For this review, take the finished solid that the model builds, in its own axes (mm). A direction names the side the tool comes from. Coordinates: 2 decimals unless noted, no trailing zeros. Write each loop counter-clockwise with the first axis right and the second up, starting at its lowest first coordinate (ties: lowest second). Pieces come first, ordered by that corner, then holes.
1) Insertion check: P1, Ø6, axis at x = 13.5, y = 476, coming from the -Z side; P2, Ø4, axis at x = 1.5, y = 165.5, coming from the -Z side; P3, Ø3.5, axis at y = 117.48, z = -28.98, coming from the -X side; P4, Ø5.5, axis at x = 91, z = -25, coming from the -Y side. Each pin has a flat end and moves straight along its axis. Give the tip position at first contact, or say it passes through.
2) We need section A-A on y = 508. Write out the cut boundary in (x, z), then the cut area to 3 significant figures.
3) We need section C-C on x = 23. Write out the cut boundary in (y, z).
4) To check wall thickness, follow line 1 along Y through (x, z) = (64, -3); line 2 along Z through (x, y) = (53, 351); line 3 along X through (y, z) = (61.5, -31). State the ranges of each line that lie inside material, in increasing order.
5) For faces 4 (the face through (95, 603.25, -16)), 5 (the face through (94.4, 358.6, -24.9)), 6 (the face through (51, 609.6, -2)), 7 (the face through (97.028, 59, -20)), list the 3-axis set-ups (+Z, -Z, +X, -X, +Y, -Y) from which the entire face can be reached by the end or side of a thin tool; tool diameter is ignored.
6) Mouldability with a two-part tool opening along X and no side actions: class faces 1 (the face through (52, 368, 0)), 2 (the face through (7.13, 358.57, -25.31)), 3 (the face through (0, 301, -20)) as pulls with the +X half, pulls with the -X half, needs draft (parallel to the pull), parting line crosses it, or undercut.
7) We need section B-B on y = 223.5. Write out the cut boundary in (x, z), then the cut area to 3 significant figures.
from build123d import *

# Parameters (mm, degrees)
BOSS_EXTRUDE1_DEPTH = 609.6
SKETCH5_W           = 92.456
SKETCH5_H           = 40.132
CUT_EXTRUDE4_DEPTH  = 94.488
SKETCH6_R           = 3.0734
SKETCH6_W           = 45.116342256
SKETCH6_H           = 16.485642943
SKETCH6_W_2         = 12.7
SKETCH6_H_2         = 20.2565
CUT_EXTRUDE5_DEPTH  = 620.310340156
SKETCH4_R           = 4.064
SKETCH4_W           = 3.175
SKETCH4_H           = 82.55
SKETCH4_R_2         = 1.524
CUT_EXTRUDE3_DEPTH  = 620.310340156
SKETCH7_W           = 92.456
SKETCH7_H           = 35.3314
CUT_EXTRUDE6_DEPTH  = 6.35
SKETCH8_W           = 92.456
SKETCH8_H           = 35.3314
CUT_EXTRUDE7_DEPTH  = 26.162
SKETCH10_R          = 1.1303
CUT_EXTRUDE8_DEPTH  = 12.7
CHAMFER1_SIZE       = 1.905
FILLET1_R           = 3.175


with BuildPart() as part:
    # Sketch1 → Boss-Extrude1 (new body)
    with BuildSketch(Plane(origin=(0, 0, 0), x_dir=(1, 0, 0), z_dir=(0, 1, 0))):
        with BuildLine():
            Line((0, 0), (0, 40.132))
            Line((0, 40.132), (2.032, 40.132))
            Line((2.032, 40.132), (4.572, 40.132))
            Line((4.572, 40.132), (9.758667803, 10.070937859))
            ThreePointArc((9.758667803, 10.070937859), (11.925571203, 6.293730916), (16.016209625, 4.8006))
            Line((16.016209625, 4.8006), (85.583790375, 4.8006))
            ThreePointArc((85.583790375, 4.8006), (89.674428797, 6.293730916), (91.841332197, 10.070937859))
            Line((91.841332197, 10.070937859), (97.028, 40.132))
            Line((97.028, 40.132), (99.568, 40.132))
            Line((99.568, 40.132), (101.6, 40.132))
            Line((101.6, 40.132), (101.6, 0))
            Line((101.6, 0), (0, 0))
        make_face()
    extrude(amount=BOSS_EXTRUDE1_DEPTH)

    # Sketch5 → Cut-Extrude4 (cut)
    with BuildSketch(Plane.XZ):
        with Locations((50.8, -20.066)):
            Rectangle(SKETCH5_W, SKETCH5_H)
    extrude(amount=-CUT_EXTRUDE4_DEPTH, mode=Mode.SUBTRACT)

    # Sketch6 → Cut-Extrude5 (cut, through all)
    with BuildSketch(Plane.XY):
        with Locations((39.7891, 596.796653012)):
            Circle(SKETCH6_R)
        with Locations((39.7891, 556.283653012)):
            Circle(SKETCH6_R)
        with Locations((61.8109, 556.283653012)):
            Circle(SKETCH6_R)
        with Locations((61.8109, 596.796653012)):
            Circle(SKETCH6_R)
        with Locations((50.8, 102.730821472)):
            Rectangle(SKETCH6_W, SKETCH6_H)
        with Locations((77.5081, 586.668403012)):
            Rectangle(SKETCH6_W_2, SKETCH6_H_2)
    extrude(amount=-CUT_EXTRUDE5_DEPTH, mode=Mode.SUBTRACT)

    # Sketch4 → Cut-Extrude3 (cut, through all)
    with BuildSketch(Plane.ZY):
        with BuildLine():
            Line((-25.208591254, 24.104081866), (-25.208591254, 29.184081866))
            ThreePointArc((-25.208591254, 29.184081866), (-29.971091254, 33.946581866), (-34.733591254, 29.184081866))
            Line((-34.733591254, 29.184081866), (-34.733591254, 24.104081866))
            ThreePointArc((-34.733591254, 24.104081866), (-29.971091254, 19.341581866), (-25.208591254, 24.104081866))
        make_face()
        with Locations((-20.066, 69.088)):
            Circle(SKETCH4_R)
        with Locations((-38.5445, 155.575)):
            Rectangle(SKETCH4_W, SKETCH4_H)
        with Locations((-38.5445, 320.675)):
            Rectangle(SKETCH4_W, SKETCH4_H)
        with Locations((-38.5445, 485.775)):
            Rectangle(SKETCH4_W, SKETCH4_H)
        with Locations(Location((-28.9814, 117.475, 0), (0, 0, 180))):
            Circle(SKETCH4_R_2)
        with Locations((-11.1506, 117.475)):
            Circle(SKETCH4_R_2)
        with Locations(Location((-11.1506, 606.425, 0), (0, 0, 315.108108431))):
            Circle(SKETCH4_R_2)
        with Locations((-28.9814, 606.425)):
            Circle(SKETCH4_R_2)
    extrude(amount=-CUT_EXTRUDE3_DEPTH, mode=Mode.SUBTRACT)

    # Sketch7 → Cut-Extrude6 (cut)
    with BuildSketch(Plane(origin=(0, 609.6, 0), x_dir=(1, 0, 0), z_dir=(0, 1, 0))):
        with Locations((50.8, 22.4663)):
            Rectangle(SKETCH7_W, SKETCH7_H)
    extrude(amount=-CUT_EXTRUDE6_DEPTH, mode=Mode.SUBTRACT)

    # Sketch8 → Cut-Extrude7 (cut)
    with BuildSketch(Plane.XZ.offset(-94.488)):
        with Locations((50.8, -22.4663)):
            Rectangle(SKETCH8_W, SKETCH8_H)
    extrude(amount=-CUT_EXTRUDE7_DEPTH, mode=Mode.SUBTRACT)

    # Sketch10 → Cut-Extrude8 (cut)
    with BuildSketch(Plane(origin=(0, 0, -36.957), x_dir=(-1, 0, 0), z_dir=(0, 0, -1))):
        with Locations((-2.286, 155.321)):
            Circle(SKETCH10_R)
        with Locations((-2.286, 320.421)):
            Circle(SKETCH10_R)
        with Locations((-2.286, 485.64141222)):
            Circle(SKETCH10_R)
        with Locations((-99.314, 155.321)):
            Circle(SKETCH10_R)
        with Locations((-99.314, 320.421)):
            Circle(SKETCH10_R)
        with Locations((-99.314, 485.64141222)):
            Circle(SKETCH10_R)
    extrude(amount=-CUT_EXTRUDE8_DEPTH, mode=Mode.SUBTRACT)

    # Chamfer1
    # the kernel refuses this chamfer: 1.905 mm, written as the material it takes off along each edge
    with BuildSketch(Plane(origin=(0, 117.475, -28.9814), x_dir=(0, 0, -1), z_dir=(0, 1, 0))) as chamfer1_piece_1:
        Polygon((1.524, -CHAMFER1_SIZE), (1.524 + CHAMFER1_SIZE, 0), (1.524, 0), align=None)
    revolve(axis=Axis((0, 117.475, -28.9814), (-1, 0, 0)), mode=Mode.SUBTRACT)
    with BuildSketch(Plane(origin=(101.6, 117.475, -28.9814), x_dir=(0, 0, -1), z_dir=(0, 1, 0))) as chamfer1_piece_2:
        Polygon((1.524, CHAMFER1_SIZE), (1.524 + CHAMFER1_SIZE, 0), (1.524, 0), align=None)
    revolve(axis=Axis((101.6, 117.475, -28.9814), (-1, 0, 0)), mode=Mode.SUBTRACT)
    with BuildSketch(Plane(origin=(101.6, 117.475, -11.1506), x_dir=(0, 0, 1), z_dir=(0, -1, 0))) as chamfer1_piece_3:
        Polygon((1.524, CHAMFER1_SIZE), (1.524 + CHAMFER1_SIZE, 0), (1.524, 0), align=None)
    revolve(axis=Axis((101.6, 117.475, -11.1506), (-1, 0, 0)), mode=Mode.SUBTRACT)
    with BuildSketch(Plane(origin=(0, 117.475, -11.1506), x_dir=(0, 0, 1), z_dir=(0, -1, 0))) as chamfer1_piece_4:
        Polygon((1.524, -CHAMFER1_SIZE), (1.524 + CHAMFER1_SIZE, 0), (1.524, 0), align=None)
    revolve(axis=Axis((0, 117.475, -11.1506), (-1, 0, 0)), mode=Mode.SUBTRACT)
    with BuildSketch(Plane(origin=(0, 606.425, -11.1506), x_dir=(0, -0.7057713201939051, 0.7084397247414577), z_dir=(0, -0.7084397247414577, -0.7057713201939051))) as chamfer1_piece_5:
        Polygon((1.524, -CHAMFER1_SIZE), (1.524 + CHAMFER1_SIZE, 0), (1.524, 0), align=None)
    revolve(axis=Axis((0, 606.425, -11.1506), (-1, 0, 0)), mode=Mode.SUBTRACT)
    with BuildSketch(Plane(origin=(101.6, 606.425, -11.1506), x_dir=(0, -0.7057713201939051, 0.7084397247414577), z_dir=(0, -0.7084397247414577, -0.7057713201939051))) as chamfer1_piece_6:
        Polygon((1.524 + CHAMFER1_SIZE, 0), (1.524, CHAMFER1_SIZE), (1.524, 0), align=None)
    revolve(axis=Axis((101.6, 606.425, -11.1506), (-1, 0, 0)), mode=Mode.SUBTRACT)
    with BuildSketch(Plane(origin=(101.6, 606.425, -28.9814), x_dir=(0, 0, 1), z_dir=(0, -1, 0))) as chamfer1_piece_7:
        Polygon((1.524 + CHAMFER1_SIZE, 0), (1.524, CHAMFER1_SIZE), (1.524, 0), align=None)
    revolve(axis=Axis((101.6, 606.425, -28.9814), (-1, 0, 0)), mode=Mode.SUBTRACT)
    with BuildSketch(Plane(origin=(0, 606.425, -28.9814), x_dir=(0, 0, 1), z_dir=(0, -1, 0))) as chamfer1_piece_8:
        Polygon((1.524, -CHAMFER1_SIZE), (1.524 + CHAMFER1_SIZE, 0), (1.524, 0), align=None)
    revolve(axis=Axis((0, 606.425, -28.9814), (-1, 0, 0)), mode=Mode.SUBTRACT)

    # Fillet1
    fillet1_edges = [part.edges().sort_by_distance(p)[0] for p in [
        (28.241828872, 110.973642943, -2.4003),
        (73.358171128, 110.973642943, -2.4003),
    ]]
    fillet(fillet1_edges, radius=FILLET1_R)


solid = part.part
Result:
1. P1: stops at z = -8.01
1. P2: stops at z = -36.96
1. P3: stops at x = 1.67
1. P4: passes through
2. outline: (0, -36.96) - (5.12, -36.96) - (9.76, -10.07) arc R6.35 cw to (16.02, -4.8) - (85.58, -4.8) arc R6.35 cw to (91.84, -10.07) - (96.48, -36.96) - (101.6, -36.96) - (101.6, 0) - (0, 0) - close
2. area: 1,010 mm2
3. outline: (94.49, -4.8) - (609.6, -4.8) - (609.6, 0) - (94.49, 0) - close
4. line 1: y = 110.97 to 554.13, 558.44 to 594.64, 598.95 to 609.6
4. line 2: z = -4.8 to 0
4. line 3: x = 0 to 4.57, 97.03 to 101.6
5. face 4: -Z, +Y
5. face 5: -Z, +Y, -Y
5. face 6: +Z, -Z, +X, -X, +Y
5. face 7: -Z, -Y
6. face 1: needs draft
6. face 2: undercut
6. face 3: pulls with the -X half
7. outline: (0, -40.13) - (4.57, -40.13) - (9.76, -10.07) arc R6.35 cw to (16.02, -4.8) - (85.58, -4.8) arc R6.35 cw to (91.84, -10.07) - (97.03, -40.13) - (101.6, -40.13) - (101.6, 0) - (0, 0) - close
7. area: 1,040 mm2
